```python
from build123d import *

# Parameters (mm, degrees)
F0_W     = 1930.4
F0_H     = 1028.7
F1_DEPTH = 12.7
F2_W     = 12.7
F2_H     = 1028.7
F2_H_2   = 927.1
F3_DEPTH = 304.8
F4_W     = 1930.4
F4_H     = 1028.7
F5_DEPTH = 12.7
F6_W     = 1930.4
F6_H     = 330.2
F7_DEPTH = 12.7


with BuildPart() as f1:
    # F0 (on Top) → F1 (new body)
    with BuildSketch(Plane.XY):
        with Locations((965.2, 514.35)):
            Rectangle(F0_W, F0_H)
    extrude(amount=F1_DEPTH)

    # F2 (on face) → F3 (join)
    with BuildSketch(Plane.XY.offset(12.7)):
        with Locations((6.35, 514.35)):
            Rectangle(F2_W, F2_H)
        with Locations((1924.05, 514.35)):
            Rectangle(F2_W, F2_H)
        with Locations((645.414, 565.15)):
            Rectangle(F2_W, F2_H_2)
        with Locations((1284.478, 565.15)):
            Rectangle(F2_W, F2_H_2)
    extrude(amount=F3_DEPTH)

    # F4 (on face) → F5 (join)
    with BuildSketch(Plane.XY.offset(317.5)):
        with Locations((965.2, 514.35)):
            Rectangle(F4_W, F4_H)
    extrude(amount=F5_DEPTH)

    # F6 (on face) → F7 (join)
    with BuildSketch(Plane(origin=(0, 1028.7, 0), x_dir=(-1, 0, 0), z_dir=(0, 1, 0))):
        with Locations((-965.2, 165.1)):
            Rectangle(F6_W, F6_H)
    extrude(amount=-F7_DEPTH)


solid = f1.part
```
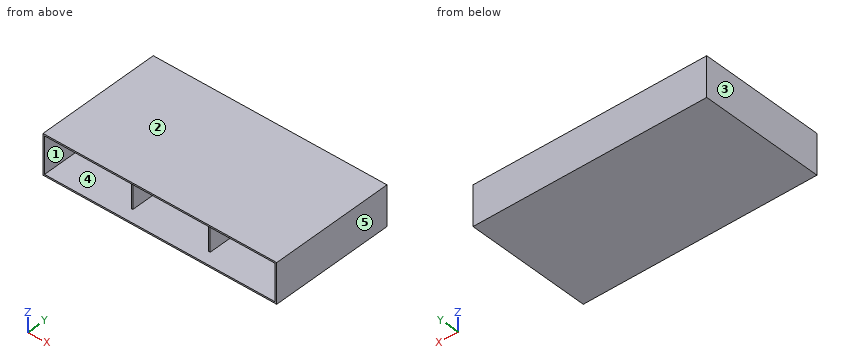
Source: CAD feature listing. Evaluate the final solid. Frame: model axes, mm. Face numbers are marked on the shaded views. A direction names the side the tool comes from. Coordinates: 2 decimals unless noted, no trailing zeros. Loops run counter-clockwise (first coordinate to the right, second up) from the corner with the lowest first, then second, coordinate; pieces in that order, holes last. Notation, with made-up numbers: M 83.5,50 L 95.5,50 A27 cw 95.5,70 Z; hole C 73,78.5 d3. An arc over 180 degrees is marked long. Put each result on its own line as item: value. Start each with the question number.
1) Ray query, L1, parallel to X at y = 899, z = 311.5; L2, parallel to Z at x = 1191.5, y = 508; L3, parallel to Y at x = 1527, z = 315. Return the intervals inside material, ascending. Write a range as from..to.
2) Reachability of the marked faces 4 and 5 from +Z, -Z, +X, -X, +Y, -Y: full face, straight path, thin tool, end or side. Return the list, or none.
3) Pull-direction query (Z, two-part tool) for the marked faces 1, 2 and 3; classes: pulls with the +Z half, pulls with the -Z half, needs draft (parallel to the pull), parting line crosses it, or undercut.
4) Contact query for flat-ended pins moving along their axis: pin 1 Ø3 at (x, z) = (874.5, 108) entering from -Y; pin 2 Ø14 at (x, z) = (1284, 148.5) entering from -Y. Output: stop coordinate, or through.
5) Cut plane C-C on x = 1795. Return the cut outline in (y, z), then the cut area to 3 significant figures.
6) Cut plane A-A on y = 597.5. Return the cut outline in (x, z), then the cut area to 3 significant figures.
7) Cut plane B-B on z = 279.5. Return the cut outline in (x, y), then the cut area to 3 significant figures.
The answers:
1. L1: x = 0..12.7, 639.06..651.76, 1278.13..1290.83, 1917.7..1930.4
1. L2: z = 0..12.7, 317.5..330.2
1. L3: y = 1016..1028.7
2. face 4: -Y
2. face 5: +Z, -Z, +X, +Y, -Y
3. face 1: undercut
3. face 2: pulls with the +Z half
3. face 3: needs draft
4. pin 1: stops at y = 1016
4. pin 2: stops at y = 101.6
5. outline: M 0,0 L 1028.7,0 L 1028.7,330.2 L 0,330.2 L 0,317.5 L 1016,317.5 L 1016,12.7 L 0,12.7 Z
5. area: 30,000 mm²
6. outline: M 0,0 L 1930.4,0 L 1930.4,330.2 L 0,330.2 Z; hole M 12.7,12.7 L 639.06,12.7 L 639.06,317.5 L 12.7,317.5 Z; hole M 651.76,12.7 L 1278.13,12.7 L 1278.13,317.5 L 651.76,317.5 Z; hole M 1290.83,12.7 L 1917.7,12.7 L 1917.7,317.5 L 1290.83,317.5 Z
6. area: 64,500 mm²
7. outline: M 0,0 L 12.7,0 L 12.7,1016 L 639.06,1016 L 639.06,101.6 L 651.76,101.6 L 651.76,1016 L 1278.13,1016 L 1278.13,101.6 L 1290.83,101.6 L 1290.83,1016 L 1917.7,1016 L 1917.7,0 L 1930.4,0 L 1930.4,1028.7 L 0,1028.7 Z
7. area: 73,500 mm²
